Autodesk Inventor part; units mm, degrees
ref_plane "YZ Plane" through (0, 0, 0) normal (1, 0, 0) x (0, 1, 0)
ref_plane "XZ Plane" through (0, 0, 0) normal (0, 1, 0) x (-1, 0, 0)
ref_plane "XY Plane" through (0, 0, 0) normal (0, 0, 1) x (1, 0, 0)
sketch "Sketch1" plane through (0, 0, 0) normal (0, 0, 1) x (1, 0, 0)
  circle A0 centre (0, 0) radius 11
  dimension "d0" = 22
extrude "Extrusion1" add sketch "Sketch1" along normal blind 3.5
sketch "Sketch2" plane through (0, 0, 3.5) normal (0, 0, 1) x (1, 0, 0)
  circle A0 centre (0, 0) radius 5
  circle A1 centre (0, 0) radius 4
  dimension "d3" = 10
  dimension "d4" = 8
extrude "Extrusion2" add sketch "Sketch2" along normal blind 10
sketch "Sketch3" plane through (0, 0, 3.5) normal (0, 0, 1) x (1, 0, 0)
  circle A0 centre (0, 0) radius 4
  dimension "d7" = 8
extrude "Extrusion3" cut sketch "Sketch3" against normal blind 10
sketch "Sketch4" plane through (0, 0, 0) normal (0, 0, -1) x (-1, 0, 0)
  circle A0 centre (0, 0) radius 4
  circle A1 centre (0, 0) radius 5
  dimension "d10" = 10
extrude "Extrusion4" add sketch "Sketch4" along normal blind 2
fillet "Fillet1" radius 0.5 1 edges at (-5, 0, 3.5)
chamfer "Chamfer1" distance 0.25 angle 45 1 edges at (-5, 0, 13.5)
chamfer "Chamfer2" distance 0.25 angle 45 2 edges at (-11, 0, 3.5) (-11, 0, 0)
sketch "Sketch5" plane through (0, 0, 3.5) normal (0, 0, 1) x (1, 0, 0)
  circle A0 centre (0, 0) radius 11 construction
  circle A1 centre (0, 0) radius 7.5 construction
  circle A2 centre (0, 7.5) radius 1.5 construction
  circle A3 centre (0, 7.5) radius 1.5
  circle A4 centre (-7.5, 0) radius 1.5 construction
  circle A5 centre (-7.5, 0) radius 1.5
  circle A6 centre (0, -7.5) radius 1.5 construction
  circle A7 centre (0, -7.5) radius 1.5
  circle A8 centre (7.5, 0) radius 1.5 construction
  circle A9 centre (7.5, 0) radius 1.5
  dimension "d21" = 15
  dimension "d20" = 22
  dimension "d22" = 3
  dimension "d25" = 360
extrude "Extrusion5" cut sketch "Sketch5" against normal through all
thread "Thread1"
properties part number "Tuerca_Tornillo de potencia"
Part model, mm, in its own coordinate system. A direction names the side the tool comes from. Coordinates: 2 decimals unless noted, no trailing zeros. Order: outer loops, then holes, each group sorted by start corner. A loop starts at its lowest first (then second) coordinate and runs counter-clockwise, first axis right, second up. Notation, with made-up numbers: (55, 2.5) -> (67, 2.5) arc R24 cw to (67, 25.5) -> close; hole circle Ø6 at (-35, -40). An arc over 180 degrees is marked (long way). Put each result on its own line as item: value. Start each with the question number.
(1) Pin check, flat tips, straight feed: pin 1 Ø10 at (x, y) = (-3, -0.5) entering from +Z; pin 2 Ø3.5 at (x, y) = (-7.5, 0) entering from -Z; pin 3 Ø3 at (x, y) = (-5.5, 4) entering from +Z; pin 4 Ø8 at (y, z) = (5.5, 5.5) entering from -X. Stop position of each tip, or through.
(2) Band-saw the part on A-A (x = 0). Count the separate pieces of the cut face and the enclosed holes in it, then the cut area to 3 significant figures.
(3) Mould opens along Y. For faces 3 (the face through (0, 4, 6)), 4 (the face through (2, -5, 0)), 5 (the face through (1.08, 4.88, -0.99)), 6 (the face through (0, 6, 2)) say: pulls with the +Y half, pulls with the -Y half, needs draft (parallel to the pull), parting line crosses it, or undercut.
(4) Which spindle directions (+Z, -Z, +X, -X, +Y, -Y) get a long thin tool onto all of the face, cutting with end or side? Do faces 1 (the face through (-2.38, 10.74, 1.73)), 2 (the face through (-1.08, 4.88, 8.56)). Say none if no direction does.
(5) Band-saw the part on C-C (z = 11.25). Give the cut face in (x, y).
(6) Probe line 1 along Y through (x, z) = (0, 1.6); line 2 along Z through (x, y) = (-4, 9.5); line 3 along Y through (x, z) = (7.5, 2.6). List the from-to ranges inside material, lowest first. Write a range as [from, to].
(7) Band-saw the part on B-B (z = 1.25). Give the cut face in (x, y).
Determined:
1. pin 1: stops at z = 13.5
1. pin 2: stops at z = 0
1. pin 3: stops at z = 3.54
1. pin 4: stops at x = -10.78
2. separate pieces: 4
2. enclosed holes: 0
2. area: 51.9 mm²
3. face 3: undercut
3. face 4: needs draft
3. face 5: parting line crosses it
3. face 6: undercut
4. face 1: +Z, -Z
4. face 2: +Z
5. outline: circle Ø10 at (0, 0); hole circle Ø8 at (0, 0)
6. line 1: y = [-11, -9], [-6, -4], [4, 6], [9, 11]
6. line 2: z = [0, 3.5]
6. line 3: y = [-8.05, -1.5], [1.5, 8.05]
7. outline: circle Ø22 at (0, 0); hole circle Ø3 at (-7.5, 0); hole circle Ø8 at (0, 0); hole circle Ø3 at (0, -7.5); hole circle Ø3 at (0, 7.5); hole circle Ø3 at (7.5, 0)
